Can you work these out from the model? Positions are in its coordinate system, mm. A direction names the side the tool comes from. Give positions to 0.01 mm unless a question says otherwise; leave off trailing zeros. Write each loop counter-clockwise with the first axis right and the second up, starting at its lowest first coordinate (ties: lowest second). Pieces come first, ordered by that corner, then holes.
1. On a 3-axis mill with a long thin cutter (end or side, diameter ignored), from which of +Z, -Z, +X, -X, +Y, -Y can I reach the whole of each face in a straight line? I mean faces 1 (the flat face through (14, 24, 3)), 2 (the flat face through (13, 24, 0)). Say none if no direction works.
2. Suppose I cut it at C-C (z = 7.25). Please give me the cut outline in (x, y) (3 decimals).
3. Suppose I cut it at A-A (y = 42.5). Please give me the cut outline in (x, z), and give its area (3 significant figures).
4. I'm going to push flat-ended pins straight in: pin 1 (2.5 mm diameter, centred on y = 30.5, z = 5.5, fed in from +X); pin 2 (1.5 mm diameter, centred on x = 12.5, z = 5, fed in from +Y); pin 3 (1 mm diameter, centred on x = 9.5, y = 20.5, fed in from -Z); pin 4 (12 mm diameter, centred on x = 13.5, y = 27.5, fed in from +Z). Where does each tip first touch, or does it pass through?
5. Suppose I cut it at B-B (x = 15.75). Please give me the cut outline in (y, z) (3 decimals).
6. If I drill on probe 1 along X at (y, z) = (44.5, 3.25), over which ranges is the centre line in solid material (lowest first)?
```python
from build123d import *

# Parameters (mm, degrees)
F0_W     = 3
F0_H     = 47.625
F0_W_2   = 22.4
F1_DEPTH = 3
F2_DEPTH = 8


with BuildPart() as f1:
    # F0 (on Top) → F1 (new body)
    with BuildSketch(Plane.XY):
        with Locations((1.5, 23.8125)):
            Rectangle(F0_W, F0_H)
        with Locations((14.2, 23.8125)):
            Rectangle(F0_W_2, F0_H)
    extrude(amount=F1_DEPTH)

    # F0 (on Top) → F2 (join)
    with BuildSketch(Plane.XY):
        with Locations((1.5, 23.8125)):
            Rectangle(F0_W, F0_H)
    extrude(amount=F2_DEPTH)


solid = f1.part
```
Checks:
1. face 1: +Z, +X, +Y, -Y
1. face 2: -Z, +X, -X, +Y, -Y
2. outline: (0, 0) - (3, 0) - (3, 47.625) - (0, 47.625) - close
3. outline: (0, 0) - (25.4, 0) - (25.4, 3) - (3, 3) - (3, 8) - (0, 8) - close
3. area: 91.2 mm2
4. pin 1: stops at x = 3
4. pin 2: passes through
4. pin 3: stops at z = 0
4. pin 4: stops at z = 3
5. outline: (0, 0) - (47.625, 0) - (47.625, 3) - (0, 3) - close
6. probe 1: x = 0 to 3
